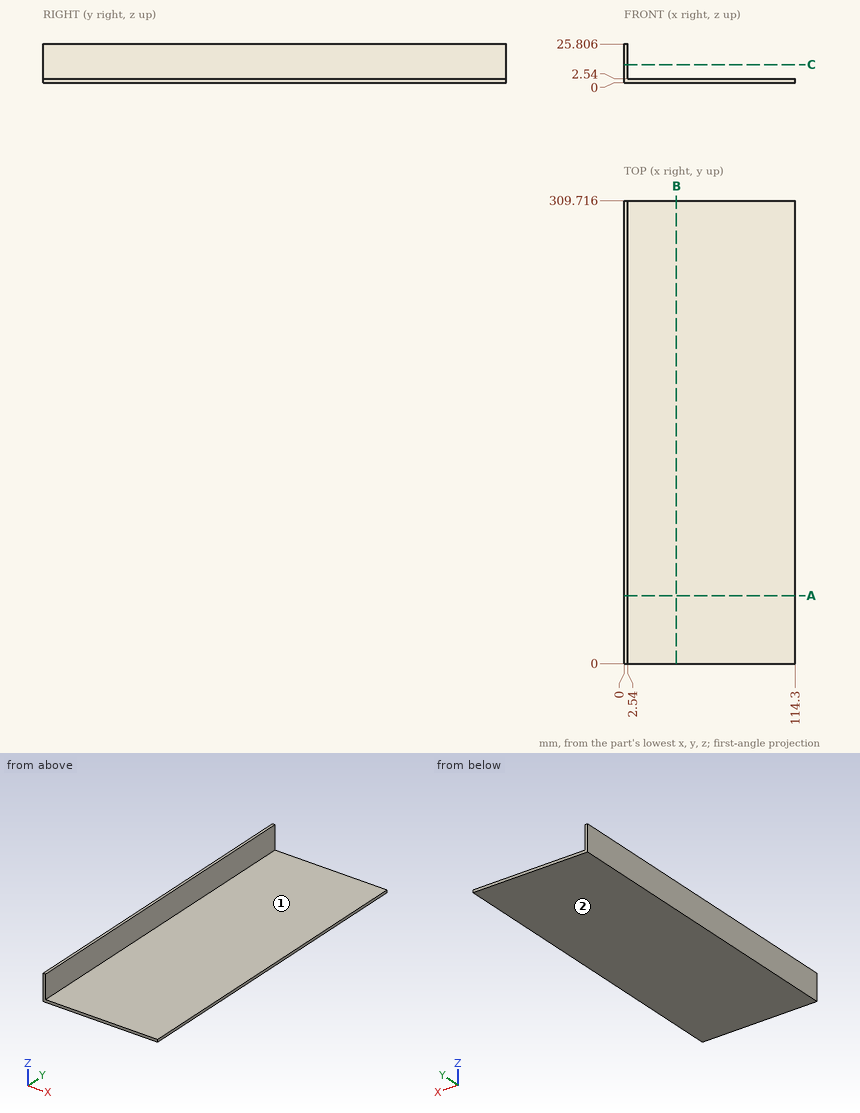
Drawing for the job (mm, zero at the part's lowest x, y, z). A direction names the side the tool comes from. Round coordinates to 2 decimals unless told otherwise and drop trailing zeros. Loops run counter-clockwise (first coordinate to the right, second up) from the corner with the lowest first, then second, coordinate; pieces in that order, holes last. Notation, with made-up numbers: (65.25, -23.75) -> (112.25, -23.75) arc R23 cw to (112.25, 7.25) -> close; hole circle Ø5 at (49.5, -2). An arc over 180 degrees is marked (long way). Use one line per item in the form item = value. Start each with the question number.
Item 1: Band-saw the part on B-B (x = 35). List the corners of the cut face in (y, z), plus the area to 3 significant figures.
Item 2: Drop flat-ended pins along their axis: pin 1 Ø1.5 at (x, y) = (18, 254) entering from +Z; pin 2 Ø11.5 at (y, z) = (207.5, 17.5) entering from +X. Give the stop position or say it passes through.
Item 3: Band-saw the part on C-C (z = 12). List the corners of the cut face in (x, y), plus the area to 3 significant figures.
Item 4: Drill centre line: line 1 along X through (y, z) = (267, 13). Where is it in solid material? Low to high.
Item 5: Band-saw the part on A-A (y = 45.5). List the corners of the cut face in (x, z).
Item 6: Tool access for the marked faces 1 and 2: list every direction of +Z, -Z, +X, -X, +Y, -Y with a clear straight run to the whole face (end or side of a thin tool).
Data:
q1.outline = (0, 0) -> (309.72, 0) -> (309.72, 2.54) -> (0, 2.54) -> close
q1.area = 787 mm^2
q2.pin_1 = 2.54
q2.pin_2 = 2.54
q3.outline = (0, 0) -> (2.54, 0) -> (2.54, 309.72) -> (0, 309.72) -> close
q3.area = 787 mm^2
q4.line_1 = 0 to 2.54
q5.outline = (0, 0) -> (114.3, 0) -> (114.3, 2.54) -> (2.54, 2.54) -> (2.54, 25.81) -> (0, 25.81) -> close
q6.face_1 = +Z, +X, +Y, -Y
q6.face_2 = -Z, +X, -X, +Y, -Y
